```python
from build123d import *

# Parameters (mm, degrees)
F0_W     = 30
F0_H     = 20
F1_DEPTH = 15
F2_W     = 15
F2_H     = 2.5
F3_DEPTH = 15.001
F4_W     = 10
F4_H     = 10
F5_DEPTH = 20.001


with BuildPart() as f1:
    # F0 (on Front) → F1 (new body)
    with BuildSketch(Plane.XZ):
        with Locations((15, 10)):
            Rectangle(F0_W, F0_H)
    extrude(amount=F1_DEPTH)

    # F2 (on Front) → F3 (cut, through all)
    with BuildSketch(Plane.XZ):
        with Locations((12.5, 1.25)):
            Rectangle(F2_W, F2_H)
        Polygon((30, 20), (15, 20), (30, 7.5), align=None)
    extrude(amount=F3_DEPTH, mode=Mode.SUBTRACT)

    # F4 (on Top) → F5 (cut, through all)
    with BuildSketch(Plane.XY):
        with Locations((25, -7.5)):
            Rectangle(F4_W, F4_H)
    extrude(amount=F5_DEPTH, mode=Mode.SUBTRACT)


solid = f1.part
```
Verification items for the finished model (mm, model axes). A direction names the side the tool comes from. Give positions to 0.01 mm unless a question says otherwise; leave off trailing zeros. Order: outer loops, then holes, each group sorted by start corner. A loop starts at its lowest first (then second) coordinate and runs counter-clockwise, first axis right, second up. Notation, with made-up numbers: (-26, -22.5) - (28, -22.5) arc R31 cw to (28, 5.5) - close; hole circle Ø4 at (22.25, 38). An arc over 180 degrees is marked (long way). Answer as CSV lines item,"result". Start each with the question number.
Item 1: Access from +Z, -Z, +X, -X, +Y, -Y to the whole of each face (thin tool, end or side, straight path). Record for faces 1 (the face through (25, -2.5, 6)), 2 (the face through (0, -7, 10)), 3 (the face through (20, -1, 1)).
Item 2: Material ranges on L1, parallel to Y at x = 23.5, z = 8.75; L2, parallel to X at y = -7, z = 3.25; L3, parallel to Z at x = 7.25, y = -6, recorded low to high.
Item 3: Gauge pin test, flat ends, axial feed: pin 1 (3 mm diameter, centred on y = -7, z = 0.5, fed in from +X); pin 2 (5 mm diameter, centred on y = -2, z = 13, fed in from +X); pin 3 (4 mm diameter, centred on x = 16, y = -5.5, fed in from -Z). Record the tip position at first contact, or that the pin passes through.
Item 4: Mould release check, pull along Y, two halves, no side actions. Record for faces 4 (the face through (11, 0, 10)), 5 (the face through (25, -12.5, 6)), 6 (the face through (11, -15, 10)), 7 (the face through (20, -8, 9)): released by +Y, released by -Y, zero draft, split by the parting line, or undercut.
Item 5: Section check C-C, the plane y = -7.75. Record the boundary of the cut face in (x, z), plus the area to 3 significant figures.
Item 6: Section check D-D, the plane z = 15.25. Record the boundary of the cut face in (x, y).
Item 7: Section check A-A, the plane x = 21. Record the boundary of the cut face in (y, z).
Item 8: Section check B-B, the plane z = 6.25. Record the boundary of the cut face in (x, y).
Filled in:
1,face 1,"+Z, -Z, +X"
1,face 2,"+Z, -Z, -X, +Y, -Y"
1,face 3,"-Z, +Y, -Y"
2,L1,"-15 to -12.5, -2.5 to 0"
2,L2,"0 to 20"
2,L3,"2.5 to 20"
3,pin 1,"x = 5"
3,pin 2,"x = 26.4"
3,pin 3,"z = 2.5"
4,face 4,"released by +Y"
4,face 5,"undercut"
4,face 6,"released by -Y"
4,face 7,"undercut"
5,outline,"(0, 0) - (5, 0) - (5, 2.5) - (20, 2.5) - (20, 15.83) - (15, 20) - (0, 20) - close"
5,area,"352 mm^2"
6,outline,"(0, -15) - (20.7, -15) - (20.7, -12.5) - (20, -12.5) - (20, -2.5) - (20.7, -2.5) - (20.7, 0) - (0, 0) - close"
7,outline,"(-15, 0) - (-12.5, 0) - (-12.5, 15) - (-15, 15) - close; (-2.5, 0) - (0, 0) - (0, 15) - (-2.5, 15) - close"
8,outline,"(0, -15) - (30, -15) - (30, -12.5) - (20, -12.5) - (20, -2.5) - (30, -2.5) - (30, 0) - (0, 0) - close"
